The listing builds one solid part. Answer for the finished solid, in the listing's coordinates (mm). A direction names the side the tool comes from. Give positions to 0.01 mm unless a question says otherwise; leave off trailing zeros. Loops run counter-clockwise (first coordinate to the right, second up) from the corner with the lowest first, then second, coordinate; pieces in that order, holes last. Notation, with made-up numbers: M 80,37.5 L 101,37.5 A18 ccw 101,44.5 Z; hole C -14,31.25 d8. An arc over 180 degrees is marked long. Return JSON: item names as keys, results as strings.
from build123d import *

# Parameters (mm, degrees)
ESBO_O1_W                = 216
ESBO_O1_H                = 106
ESBO_O1_W_2              = 97.5
ESBO_O1_H_2              = 42.5
RESSALTO_EXTRUS_O1_DEPTH = 3
ESBO_O2_R                = 3
RESSALTO_EXTRUS_O2_DEPTH = 3
ESBO_O3_R                = 2
CORTE_EXTRUS_O1_DEPTH    = 1


with BuildPart() as part:
    # Esboço1 → Ressalto-extrusão1 (new body)
    with BuildSketch(Plane.XY):
        with Locations((-24.354637835, -10.294366601)):
            Rectangle(ESBO_O1_W, ESBO_O1_H)
        with Locations((-76.604637835, 14.455633399)):
            Rectangle(ESBO_O1_W_2, ESBO_O1_H_2, mode=Mode.SUBTRACT)
        with Locations((27.895362165, 14.455633399)):
            Rectangle(ESBO_O1_W_2, ESBO_O1_H_2, mode=Mode.SUBTRACT)
        with Locations((27.895362165, -35.044366601)):
            Rectangle(ESBO_O1_W_2, ESBO_O1_H_2, mode=Mode.SUBTRACT)
        with Locations((-76.604637835, -35.044366601)):
            Rectangle(ESBO_O1_W_2, ESBO_O1_H_2, mode=Mode.SUBTRACT)
    extrude(amount=RESSALTO_EXTRUS_O1_DEPTH)

    # Esboço2 → Ressalto-extrusão2 (add)
    with BuildSketch(Plane.XY.offset(3)):
        with Locations((-24.354637835, -10.294366601)):
            Circle(ESBO_O2_R)
    extrude(amount=RESSALTO_EXTRUS_O2_DEPTH)

    # Esboço3 → Corte-extrusão1 (cut)
    with BuildSketch(Plane(origin=(0, 0, 0), x_dir=(-1, 0, 0), z_dir=(0, 0, -1))):
        with Locations((-79.645362165, 38.705633399)):
            Circle(ESBO_O3_R)
        with Locations((128.354637835, 38.705633399)):
            Circle(ESBO_O3_R)
        with Locations((-79.645362165, -59.294366601)):
            Circle(ESBO_O3_R)
        with Locations((128.354637835, -59.294366601)):
            Circle(ESBO_O3_R)
    extrude(amount=-CORTE_EXTRUS_O1_DEPTH, mode=Mode.SUBTRACT)


solid = part.part
(1) The part is cut by section B-B (z = 2). Determine the outline of the cut face in (x, y), and give its area (3 significant figures).
Values follow:
{"outline": "M -132.35,-63.29 L 83.65,-63.29 L 83.65,42.71 L -132.35,42.71 Z; hole M -125.35,-56.29 L -27.85,-56.29 L -27.85,-13.79 L -125.35,-13.79 Z; hole M -125.35,-6.79 L -27.85,-6.79 L -27.85,35.71 L -125.35,35.71 Z; hole M -20.85,-56.29 L 76.65,-56.29 L 76.65,-13.79 L -20.85,-13.79 Z; hole M -20.85,-6.79 L 76.65,-6.79 L 76.65,35.71 L -20.85,35.71 Z", "area": "6,320 mm²"}
(2) The part is cut by section A-A (x = -30.5). Determine the outline of the cut face in (y, z).
Values follow:
{"outline": "M -63.29,0 L -56.29,0 L -56.29,3 L -63.29,3 Z; M -13.79,0 L -6.79,0 L -6.79,3 L -13.79,3 Z; M 35.71,0 L 42.71,0 L 42.71,3 L 35.71,3 Z"}
(3) Given pin 1 (2 mm diameter, centred on x = -3, y = -10, fed in from +Z); pin 2 (3 mm diameter, centred on x = -128.35, y = 38.71, fed in from -Z), each flat-ended and moving along its own axis, determine where each tip first touches the part or whether it passes through.
Values follow:
{"pin 1": "z = 3", "pin 2": "z = 1"}
(4) A tool of negligible diameter and unlimited length cuts with its end or side. For faces 4 (the flat face through (80, -59, 1)), 5 (the flat face through (-24, -10, 6)), 6 (the flat face through (-26, 2, 3)), from which of +Z, -Z, +X, -X, +Y, -Y can it reach the whole face along a straight path? Write none if from no direction.
Values follow:
{"face 4": "-Z", "face 5": "+Z, +X, -X, +Y, -Y", "face 6": "+Z"}
(5) Straight lines are drawn through the part: line 1 along Y through (x, z) = (-107, 2.5); line 2 along X through (y, z) = (-35, 1.8); line 3 along Z through (x, y) = (-23, 29.5). For each, find the intervals that lie inside material, in ascending order.
Values follow:
{"line 1": "-63.29 to -56.29, -13.79 to -6.79, 35.71 to 42.71", "line 2": "-132.35 to -125.35, -27.85 to -20.85, 76.65 to 83.65", "line 3": "0 to 3"}
(6) Determine the mould class of faces 1 (the flat face through (-26, -10, 0)), 2 (the cylindrical face through (-22.742, -7.765, 4.479)), 3 (the cylindrical face through (80.079, -61.247, 0.493)) for opening direction Y: released by +Y, released by -Y, zero draft, split by the parting line, or undercut.
Values follow:
{"face 1": "zero draft", "face 2": "split by the parting line", "face 3": "undercut"}
(7) The part is cut by section C-C (y = -35.5). Determine the outline of the cut face in (x, z).
Values follow:
{"outline": "M -132.35,0 L -125.35,0 L -125.35,3 L -132.35,3 Z; M -27.85,0 L -20.85,0 L -20.85,3 L -27.85,3 Z; M 76.65,0 L 83.65,0 L 83.65,3 L 76.65,3 Z"}
